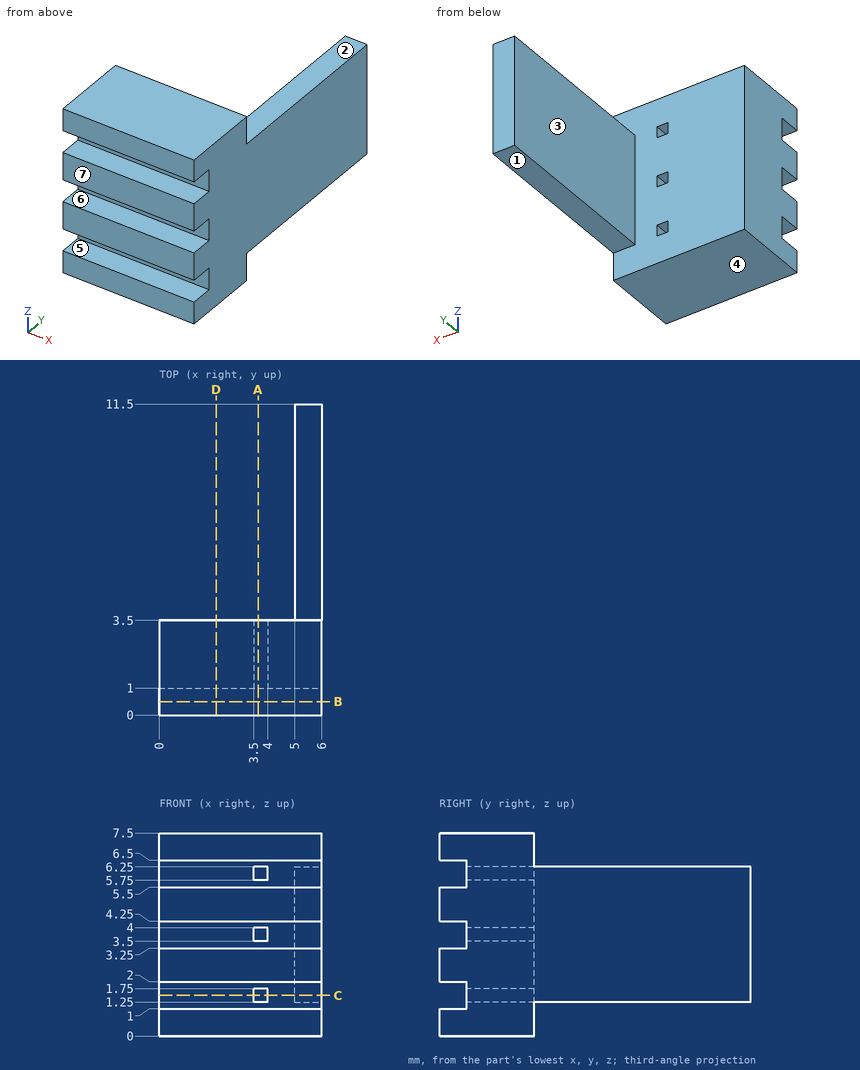
For this review, use the dimensioned drawing (mm, ordinates from the lowest corner) and the shaded views. A direction names the side the tool comes from. Round coordinates to 2 decimals unless told otherwise and drop trailing zeros. Loops run counter-clockwise (first coordinate to the right, second up) from the corner with the lowest first, then second, coordinate; pieces in that order, holes last. Notation, with made-up numbers: M 83.5,80 L 113.5,80 A18 cw 113.5,113 Z; hole C 81,-7.75 d7. An arc over 180 degrees is marked long. Answer as a JSON object with one key per item and string values.
(1) Clearance check with flat-ended pins moving along their axes: P1, Ø4, axis at y = 6, z = 3.5, coming from the -X side; P2, Ø1.5, axis at x = 5, y = 8, coming from the +Z side; P3, Ø3, axis at x = 2.5, z = 5, coming from the +Y side. State where each tip first meets the part, or that it passes through.
Resolved:
{"P1": "x = 5", "P2": "z = 6.25", "P3": "y = 3.5"}
(2) Draft analysis for pull direction Z (two halves, no side actions). For the marked faces 4, 5, 6 and 7, state which applies: released by +Z, released by -Z, zero draft, split by the parting line, or undercut.
Resolved:
{"face 4": "released by -Z", "face 5": "undercut", "face 6": "undercut", "face 7": "zero draft"}
(3) Take a section at A-A on x = 3.65. Give the boundary of the cut face in (y, z), and give its area (3 significant figures).
Resolved:
{"outline": "M 0,0 L 3.5,0 L 3.5,1.25 L 1,1.25 L 1,1 L 0,1 Z; M 0,2 L 1,2 L 1,1.75 L 3.5,1.75 L 3.5,3.5 L 1,3.5 L 1,3.25 L 0,3.25 Z; M 0,4.25 L 1,4.25 L 1,4 L 3.5,4 L 3.5,5.75 L 1,5.75 L 1,5.5 L 0,5.5 Z; M 0,6.5 L 1,6.5 L 1,6.25 L 3.5,6.25 L 3.5,7.5 L 0,7.5 Z", "area": "19.5 mm²"}
(4) Take a section at B-B on y = 0.5. Give the boundary of the cut face in (x, z), and give its area (3 significant figures).
Resolved:
{"outline": "M 0,0 L 6,0 L 6,1 L 0,1 Z; M 0,2 L 6,2 L 6,3.25 L 0,3.25 Z; M 0,4.25 L 6,4.25 L 6,5.5 L 0,5.5 Z; M 0,6.5 L 6,6.5 L 6,7.5 L 0,7.5 Z", "area": "27.0 mm²"}
(5) Take a section at C-C on z = 1.5. Give the boundary of the cut face in (x, y), and give its area (4 significant figures).
Resolved:
{"outline": "M 0,1 L 3.5,1 L 3.5,3.5 L 0,3.5 Z; M 4,1 L 6,1 L 6,11.5 L 5,11.5 L 5,3.5 L 4,3.5 Z", "area": "21.75 mm²"}
(6) Tool access review of the marked faces 1, 2 and 3: name each direction out of +Z, -Z, +X, -X, +Y, -Y from which nothing blocks a thin tool from reaching the whole face with its end or side.
Resolved:
{"face 1": "-Z, +X, -X, +Y", "face 2": "+Z, +X, -X, +Y", "face 3": "+Z, -Z, -X, +Y"}
(7) To check wall thickness, follow line 1 along Y through (x, z) = (5.35, 1.75); line 2 along X through (y, z) = (10.5, 6); line 3 along Y through (x, z) = (2, 6.25). State the ranges of each line that lie inside material, in increasing order.
Resolved:
{"line 1": "1 to 11.5", "line 2": "5 to 6", "line 3": "1 to 3.5"}
(8) Take a section at D-D on x = 2.1. Give the boundary of the cut face in (y, z).
Resolved:
{"outline": "M 0,0 L 3.5,0 L 3.5,7.5 L 0,7.5 L 0,6.5 L 1,6.5 L 1,5.5 L 0,5.5 L 0,4.25 L 1,4.25 L 1,3.25 L 0,3.25 L 0,2 L 1,2 L 1,1 L 0,1 Z"}
